Autodesk Inventor part; units mm, degrees
ref_plane "YZ Plane" through (0, 0, 0) normal (1, 0, 0) x (0, 1, 0)
ref_plane "XZ Plane" through (0, 0, 0) normal (0, 1, 0) x (-1, 0, 0)
ref_plane "XY Plane" through (0, 0, 0) normal (0, 0, 1) x (1, 0, 0)
sketch "Sketch2" plane through (0, 0, 0) normal (0, 1, 0) x (-1, 0, 0)
  circle A0 centre (0, 0) radius 8.636
  dimension "d0" = 17.272
extrude "Extrusion1" add sketch "Sketch2" against normal blind 1.778
sketch "Sketch3" plane through (0, -1.778, 0) normal (0, -1, 0) x (1, 0, 0)
  circle A0 centre (0, 0) radius 6.35
  dimension "d3" = 12.7
extrude "Extrusion2" add sketch "Sketch3" along normal blind 19.304
sketch "Sketch4" plane through (0, -21.082, 0) normal (0, -1, 0) x (1, 0, 0)
  point P0 (0, 0)
  point P1 (0, 0)
hole "Hole1" at (0, -21.082, 0) direction (0, 1, 0) diameter 8.376 end through all
sketch "Sketch5" plane through (0, 0, 0) normal (0, 1, 0) x (1, 0, 0)
  circle A0 centre (0, 0) radius 5.5499
  dimension "d13" = 11.0998
extrude "Extrusion3" cut sketch "Sketch5" against normal blind 9.1694
properties part number "M10x1_5_insert"
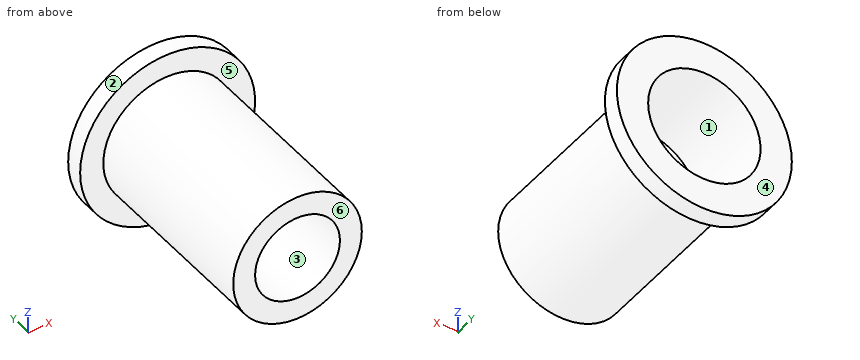
Verification items for the finished model (mm, model axes). Face numbers are marked on the shaded views. A direction names the side the tool comes from. Round coordinates to 2 decimals unless told otherwise and drop trailing zeros. Loops run counter-clockwise (first coordinate to the right, second up) from the corner with the lowest first, then second, coordinate; pieces in that order, holes last. Notation, with made-up numbers: M -40,-29.5 L -25,-29.5 A6 ccw -25,-21.5 Z; hole C 15,10.5 d3. An arc over 180 degrees is marked long. Write each question's results on one line, items separated by ' | '.
1) Section check C-C on y = -12. Record the boundary of the cut face in (x, z).
Checks:
outline: C 0,0 d12.7; hole C 0,0 d8.38
2) Gauge pin test, flat ends, axial feed: P1, Ø8, axis at y = -8, z = -5, coming from the +X side; P2, Ø2, axis at x = 6, y = -2.5, coming from the +Z side; P3, Ø1, axis at x = 3, y = -15, coming from the +Z side; P4, Ø5, axis at x = 3, z = 2.5, coming from the -Y side. Record the tip position at first contact, or that the pin passes through.
Checks:
P1: stops at x = 6.27 | P2: stops at z = 6.81 | P3: stops at z = 5.84 | P4: stops at y = -21.08
3) Section check D-D on z = 5.25. Record the boundary of the cut face in (x, y), then the cut area to 3 significant figures.
Checks:
outline: M -6.86,-1.78 L -3.57,-1.78 L -3.57,-21.08 L 3.57,-21.08 L 3.57,-1.78 L 6.86,-1.78 L 6.86,0 L 1.8,0 L 1.8,-9.17 L -1.8,-9.17 L -1.8,0 L -6.86,0 Z | area: 129 mm2
4) Scan lines: L1, parallel to Z at x = 0, y = -6; L2, parallel to Z at x = 0, y = -12; L3, parallel to Y at x = 4.5, z = -6.25. Record each from-to range of solid material in increasing order. Write a range as from..to.
Checks:
L1: z = -6.35..-5.55, 5.55..6.35 | L2: z = -6.35..-4.19, 4.19..6.35 | L3: y = -1.78..0
5) Mould release check, pull along X, two halves, no side actions. Record for the marked faces 1, 2, 3 and 4: released by +X, released by -X, zero draft, split by the parting line, or undercut.
Checks:
face 1: undercut | face 2: split by the parting line | face 3: undercut | face 4: zero draft
6) Section check A-A on z = 0. Record the boundary of the cut face in (x, y), then the cut area to 3 significant figures.
Checks:
outline: M -8.64,-1.78 L -6.35,-1.78 L -6.35,-21.08 L -4.19,-21.08 L -4.19,-9.17 L -5.55,-9.17 L -5.55,0 L -8.64,0 Z; M 4.19,-21.08 L 6.35,-21.08 L 6.35,-1.78 L 8.64,-1.78 L 8.64,0 L 5.55,0 L 5.55,-9.17 L 4.19,-9.17 Z | area: 74.3 mm2
7) Section check B-B on x = 0. Record the boundary of the cut face in (y, z).
Checks:
outline: M -21.08,-6.35 L -1.78,-6.35 L -1.78,-8.64 L 0,-8.64 L 0,-5.55 L -9.17,-5.55 L -9.17,-4.19 L -21.08,-4.19 Z; M -21.08,4.19 L -9.17,4.19 L -9.17,5.55 L 0,5.55 L 0,8.64 L -1.78,8.64 L -1.78,6.35 L -21.08,6.35 Z
8) Access from +Z, -Z, +X, -X, +Y, -Y to the whole of each face (thin tool, end or side, straight path). Record for the marked faces 5 and 6.
Checks:
face 5: -Y | face 6: +Z, -Z, +X, -X, -Y
